Input: part model. Units: mm. Frame: model coordinates. Coordinates: 2 decimals unless noted, no trailing zeros. Write each loop counter-clockwise with the first axis right and the second up, starting at its lowest first coordinate (ties: lowest second). Pieces come first, ordered by that corner, then holes. Notation, with made-up numbers: (30, -31.5) -> (67, -31.5) arc R30 cw to (67, -3.5) -> close; hole circle Ø8 at (9, 82.25). An arc over 180 degrees is marked (long way). Use one line per item in the form item = value. Start each with the question number.
(1) Pull-direction query (X, two-part tool) for faces 1 (the face through (6.7, 0.6, -33.9)), 2 (the face through (0, 1, 1)), 3 (the face through (6.7, 0.6, 35.1)); classes: released by +X, released by -X, zero draft, split by the parting line, or undercut.
(2) Ray query, line 1 along Z through (x, y) = (6.25, 0.85); line 2 along X through (y, z) = (0.7, -34.5). Return the intervals inside material, ascending.
(3) Cut plane B-B on z = 34.5. Return the cut outline in (x, y).
(4) Cut plane A-A on x = 6.25. Return the cut outline in (y, z), plus the area to 3 significant figures.
```python
from build123d import *

# Parameters (mm, degrees)
F0_W     = 18.5
F0_H     = 74
F0_R     = 1
F0_R_2   = 0.75
F1_DEPTH = 1
F2_SIZE  = 0.25


with BuildPart() as f1:
    # F0 (on Front) → F1 (new body)
    with BuildSketch(Plane.XZ):
        Rectangle(F0_W, F0_H)
        with Locations((6.25, -34.5)):
            Circle(F0_R, mode=Mode.SUBTRACT)
        with Locations((6.25, 34.5)):
            Circle(F0_R, mode=Mode.SUBTRACT)
        with Locations((6.25, -34.5)):
            Circle(F0_R)
        with Locations((6.25, -34.5)):
            Circle(F0_R_2, mode=Mode.SUBTRACT)
        with Locations((6.25, 34.5)):
            Circle(F0_R)
        with Locations((6.25, 34.5)):
            Circle(F0_R_2, mode=Mode.SUBTRACT)
    extrude(amount=-F1_DEPTH)

    # F2
    f2_edges = [f1.edges().sort_by_distance(p)[0] for p in [
        (5.5, 0, -34.5),
        (5.5, 0, 34.5),
    ]]
    chamfer(f2_edges, length=F2_SIZE)


solid = f1.part
```
Values:
q1.face_1 = undercut
q1.face_2 = zero draft
q1.face_3 = undercut
q2.line_1 = -37 to -35.25, -33.75 to 33.75, 35.25 to 37
q2.line_2 = -9.25 to 5.5, 7 to 9.25
q3.outline = (-9.25, 0) -> (5.25, 0) -> (5.5, 0.25) -> (5.5, 1) -> (-9.25, 1) -> close; (7, 0.25) -> (7.25, 0) -> (9.25, 0) -> (9.25, 1) -> (7, 1) -> close
q4.outline = (0, -37) -> (1, -37) -> (1, -35.25) -> (0.25, -35.25) -> (0, -35.5) -> close; (0, -33.5) -> (0.25, -33.75) -> (1, -33.75) -> (1, 33.75) -> (0.25, 33.75) -> (0, 33.5) -> close; (0, 35.5) -> (0.25, 35.25) -> (1, 35.25) -> (1, 37) -> (0, 37) -> close
q4.area = 70.9 mm2
